```python
from build123d import *

# Parameters (mm, degrees)
BOSS_EXTRUDE1_START = -0.65
BOSS_EXTRUDE1_DEPTH = 5
CUT_EXTRUDE1_START  = -5.65
SKETCH2_3_R         = 3
SKETCH2_3_R_2       = 2
CUT_EXTRUDE1_DEPTH  = 3.5
CUT_EXTRUDE2_START  = -2.15
SKETCH2_4_R         = 2
CUT_EXTRUDE2_DEPTH  = 1.5
CUT_EXTRUDE3_START  = -4.15
SKETCH2_5_R         = 3
CUT_EXTRUDE3_DEPTH  = 3.5
CUT_EXTRUDE4_START  = -5.65
SKETCH2_6_R         = 2
CUT_EXTRUDE4_DEPTH  = 1.5


with BuildPart() as part:
    # Sketch2 → Boss-Extrude1 (new body)
    with BuildSketch(Plane(origin=(0, 0, 0), x_dir=(0, 0, -1), z_dir=(1, 0, 0)).offset(BOSS_EXTRUDE1_START)):
        with BuildLine():
            Line((0.474149458, -9.067560136), (-12.581681775, -73.461136983))
            ThreePointArc((-12.581681775, -73.461136983), (-17.296746951, -76.586542619), (-20.422152587, -71.871477443))
            Line((-20.422152587, -71.871477443), (-7.366321354, -7.477900597))
            ThreePointArc((-7.366321354, -7.477900597), (-6.977161002, -5.987839937), (-6.425552448, -4.549975356))
            Line((-6.425552448, -4.549975356), (-3.649510541, 1.637398184))
            ThreePointArc((-3.649510541, 1.637398184), (1.637398184, 3.649510541), (3.649510541, -1.637398184))
            Line((3.649510541, -1.637398184), (0.873468634, -7.824771725))
            ThreePointArc((0.873468634, -7.824771725), (0.639332629, -8.435088345), (0.474149458, -9.067560136))
        make_face()
    extrude(amount=-BOSS_EXTRUDE1_DEPTH)

    # Sketch2<3> → Cut-Extrude1 (cut)
    # profile 1 of 2: a face of its own
    with BuildSketch(Plane(origin=(0, 0, 0), x_dir=(0, 0, -1), z_dir=(1, 0, 0)).offset(CUT_EXTRUDE1_START)):
        with Locations(Location((0, 0, 0), (0, 0, 180))):
            Circle(SKETCH2_3_R)
        Circle(SKETCH2_3_R_2, mode=Mode.SUBTRACT)
    # profile 2 of 2: a face of its own
    with BuildSketch(Plane(origin=(0, 0, 0), x_dir=(0, 0, -1), z_dir=(1, 0, 0)).offset(CUT_EXTRUDE1_START)):
        Circle(SKETCH2_3_R_2)
    extrude(amount=CUT_EXTRUDE1_DEPTH, mode=Mode.SUBTRACT)

    # Sketch2<4> → Cut-Extrude2 (cut)
    with BuildSketch(Plane(origin=(0, 0, 0), x_dir=(0, 0, -1), z_dir=(1, 0, 0)).offset(CUT_EXTRUDE2_START)):
        Circle(SKETCH2_4_R)
    extrude(amount=CUT_EXTRUDE2_DEPTH, mode=Mode.SUBTRACT)

    # Sketch2<5> → Cut-Extrude3 (cut)
    with BuildSketch(Plane(origin=(0, 0, 0), x_dir=(0, 0, -1), z_dir=(1, 0, 0)).offset(CUT_EXTRUDE3_START)):
        with Locations((-16.501917181, -72.666307213)):
            Circle(SKETCH2_5_R)
    extrude(amount=CUT_EXTRUDE3_DEPTH, mode=Mode.SUBTRACT)

    # Sketch2<6> → Cut-Extrude4 (cut)
    with BuildSketch(Plane(origin=(0, 0, 0), x_dir=(0, 0, -1), z_dir=(1, 0, 0)).offset(CUT_EXTRUDE4_START)):
        with Locations((-16.501917181, -72.666307213)):
            Circle(SKETCH2_6_R)
    extrude(amount=CUT_EXTRUDE4_DEPTH, mode=Mode.SUBTRACT)


solid = part.part
```
Read the model definition and answer for the solid it produces. Units are mm, in the model's axes. A direction names the side the tool comes from. Coordinates: 2 decimals unless noted, no trailing zeros. Order: outer loops, then holes, each group sorted by start corner. A loop starts at its lowest first (then second) coordinate and runs counter-clockwise, first axis right, second up. Notation, with made-up numbers: (3.25, -7.5) - (33.25, -7.5) arc R6 ccw to (33.25, -2.5) - close; hole circle Ø11 at (43.25, -38.5). An arc over 180 degrees is marked (long way). Answer as a JSON object with one key per item and string values. Group by question number.
Item 1: The mould has two halves that part along Y. Classify faces 4 (the face through (-5.65, -36, 7)), 5 (the face through (-4.911, -74.619, 16.935)), 6 (the face through (-3.115, -40.125, 13.986)), 7 (the face through (-3, -41, 6)): +Y half, -Y half, draft (parallel to the pull), parting line (faces both ways), or undercut.
Item 2: Section B-B (x = -2.95) is taken. Give the vertices of the cut face in (y, z).
Item 3: A flat-ended cylindrical pin translates along its axis: P1, Ø2.5, axis at y = -72.67, z = 16.5, coming from the +X side. Find the tip coordinate at first contact, or state that the pin passes through.
Item 4: Consider probe 1 along Y at (x, z) = (-1.75, -1.5); probe 2 along Z at (x, y) = (-3, -18); probe 3 along Z at (x, y) = (-5.4, -25.5). Determine where each line is inside the solid, lowest interval first. Write a range as from..to.
Item 5: Section A-A (y = 0) is taken. Give the vertices of the cut face in (x, z), plus the area to 3 significant figures.
Item 6: Section C-C (z = 17.25) is taken. Give the vertices of the cut face in (x, y).
Item 7: Section D-D (y = -27.5) is taken. Give the vertices of the cut face in (x, z).
Item 8: A tool of negligible diameter and unlimited length cuts with its end or side. For faces 1 (the face through (-3.92, -0.9, 2.86)), 2 (the face through (-4.15, -75, 16)), 3 (the face through (-3.115, -6.008, 6.984)), from which of +Z, -Z, +X, -X, +Y, -Y can it reach the whole face along a straight path? Write none if from no direction.
Results are:
{
 "1": {"face 4": "draft", "face 5": "undercut", "face 6": "+Y half", "face 7": "-Y half"},
 "2": {"outline": "(-73.46, 12.58) - (-9.07, -0.47) arc R5.9 cw to (-7.82, -0.87) - (-1.64, -3.65) arc R4 ccw to (1.64, 3.65) - (-4.55, 6.43) arc R13.9 ccw to (-7.48, 7.37) - (-71.87, 20.42) arc R4 ccw to start; hole circle Ø6 at (-72.67, 16.5); hole circle Ø6 at (0, 0)"},
 "3": {"P1": "passes through"},
 "4": {"probe 1": "y = -6.43..-1.32, 1.32..3.71", "probe 2": "z = 1.34..9.5", "probe 3": "z = 2.86..11.02"},
 "5": {"outline": "(-5.65, -4) - (-0.65, -4) - (-0.65, -2) - (-2.15, -2) - (-2.15, -3) - (-5.65, -3) - close; (-5.65, 3) - (-2.15, 3) - (-2.15, 2) - (-0.65, 2) - (-0.65, 4.38) - (-5.65, 4.38) - close", "area": "14.9 mm^2"},
 "6": {"outline": "(-5.65, -76.6) - (-0.65, -76.6) - (-0.65, -75.57) - (-4.15, -75.57) - (-4.15, -74.52) - (-5.65, -74.52) - close; (-5.65, -70.81) - (-4.15, -70.81) - (-4.15, -69.76) - (-0.65, -69.76) - (-0.65, -56.23) - (-5.65, -56.23) - close"},
 "7": {"outline": "(-5.65, 3.26) - (-0.65, 3.26) - (-0.65, 11.43) - (-5.65, 11.43) - close"},
 "8": {"face 1": "-X", "face 2": "+X", "face 3": "+Z, +X, -X, +Y"}
}
